Verification items for the finished model (mm, model axes). Face numbers are marked on the shaded views. A direction names the side the tool comes from. Round coordinates to 2 decimals unless told otherwise and drop trailing zeros. Order: outer loops, then holes, each group sorted by start corner. A loop starts at its lowest first (then second) coordinate and runs counter-clockwise, first axis right, second up. Notation, with made-up numbers: M -17.5,-2 L 21.5,-2 A16 ccw 21.5,12 Z; hole C 23.25,35.5 d5. An arc over 180 degrees is marked long. Write item = value, one per line. Start each with the question number.
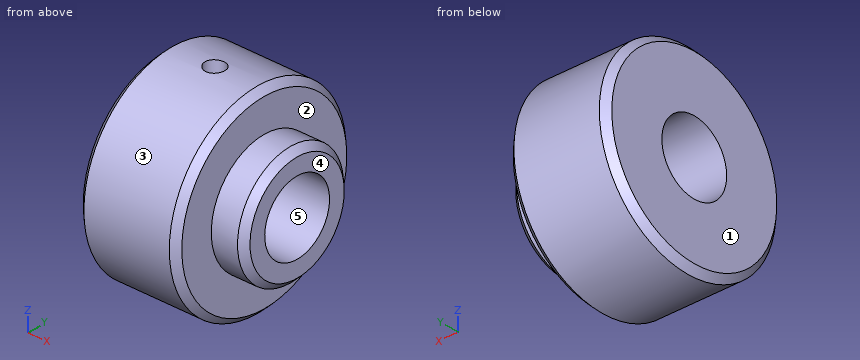
from build123d import *

# Parameters (mm, degrees)
F2_SIZE  = 2
F5_D     = 6
F5_DEPTH = 12
F5_START = 0.150377
F5_TIP   = 1.8025818571


with BuildPart() as f1:
    # F0 (on Front) → F1 (revolve)
    with BuildSketch(Plane.XZ):
        Polygon((0, 30), (-30, 30), (-30, 11), (10, 11), (10, 18), (0, 18), align=None)
    revolve(axis=Axis((3.7253e-06, 0, 0), (1, 0, 0)))

    # F2
    f2_edges = [f1.edges().sort_by_distance(p)[0] for p in [
        (0, 0, -30),
        (-30, 0, -30),
        (-15, 0, 30),
        (10, 0, -18),
    ]]
    chamfer(f2_edges, length=F2_SIZE)

    # F5
    # its depths count from where the whole tool has entered the part; down to there all is cleared
    with Locations(Plane.XY.offset(30).offset(-F5_START)):
        with Locations((-15, 0)):
            Hole(F5_D / 2, depth=F5_DEPTH)
            with Locations((0, 0, -(F5_DEPTH + F5_TIP / 2))):  # 118° drill point
                Cone(0, F5_D / 2, F5_TIP, mode=Mode.SUBTRACT)


solid = f1.part
1) Cross-section at A-A, the plane z = 0. Enter the section's corners in (x, y), then the cut area to 3 significant figures.
2) Cross-section at C-C, the plane x = -5.5. Enter the section's corners in (y, z).
3) Release check for a two-part mould opening along Y. For the marked faces 3, 4 and 5 record: pulls with the +Y half, pulls with the -Y half, needs draft (parallel to the pull), parting line crosses it, or undercut.
4) Access from +Z, -Z, +X, -X, +Y, -Y to the whole of each face (thin tool, end or side, straight path). Record for the marked faces 1 and 2.
5) Scan lines: probe 1 along X at (y, z) = (0, 24); probe 2 along Y at (x, z) = (2, -0.5); probe 3 along X at (y, z) = (19.5, 4.5). Record each from-to range of solid material in increasing order.
6) Gauge pin test, flat ends, axial feed: P1, Ø6, axis at x = -12, y = -13.5, coming from the -Z side; P2, Ø8, axis at x = 0, y = 8.5, coming from the -Z side; P3, Ø1, axis at x = -23, z = 2.5, coming from the -Y side. Record the tip position at first contact, or that the pin passes through.
7) Cross-section at B-B, the plane x = -1. Enter the section's corners in (y, z).
Geometry results:
q1.outline = M -30,-28 L -28,-30 L -2,-30 L 0,-28 L 0,-18 L 8,-18 L 10,-16 L 10,-11 L -30,-11 Z; M -30,11 L 10,11 L 10,16 L 8,18 L 0,18 L 0,28 L -2,30 L -28,30 L -30,28 Z
q1.area = 1,270 mm^2
q2.outline = C 0,0 d60; hole C 0,0 d22
q3.face_3 = parting line crosses it
q3.face_4 = needs draft
q3.face_5 = undercut
q4.face_1 = +Z, -Z, -X, +Y, -Y
q4.face_2 = +X
q5.probe_1 = -30 to -18, -12 to 0
q5.probe_2 = -17.99 to -10.99, 10.99 to 17.99
q5.probe_3 = -30 to 0
q6.P1 = -28.1
q6.P2 = -29.57
q6.P3 = -29.93
q7.outline = C 0,0 d58; hole C 0,0 d22
